Autodesk Inventor part; units mm, degrees
ref_plane "YZ Plane" through (0, 0, 0) normal (1, 0, 0) x (0, 1, 0)
ref_plane "XZ Plane" through (0, 0, 0) normal (0, 1, 0) x (-1, 0, 0)
ref_plane "XY Plane" through (0, 0, 0) normal (0, 0, 1) x (1, 0, 0)
sketch "Эскиз1" plane through (0, 0, 0) normal (0, 0, 1) x (1, 0, 0)
  line L0 (0, 0) -> (68, 0)
  line L1 (68, 0) -> (68, 35)
  line L2 (68, 35) -> (0, 35)
  line L3 (0, 35) -> (0, 0)
  line L4 (5, 30) -> (63, 30)
  line L5 (63, 30) -> (63, 3)
  line L6 (63, 3) -> (5, 3)
  line L7 (5, 3) -> (5, 30)
  line L8 (5, 3) -> (0, 3)
  line L9 (63, 3) -> (68, 3)
  dimension "d0" = 5
  dimension "d1" = 5
  dimension "d2" = 5
  dimension "d3" = 3
  dimension "d4" = 68
  dimension "d5" = 35
extrude "Выдавливание1" add sketch "Эскиз1" along normal blind 3 contours L3 L2 L1 L9 L5 L4 L7 L8
extrude "Выдавливание2" add sketch "Эскиз1" along normal blind 25 contours L3 L8 L6 L9 L1 L0
sketch "Эскиз2" plane through (0, 0, 0) normal (0, -1, 0) x (1, 0, 0)
  circle A0 centre (34, 12.5) radius 1
  line L0 (0, 0) -> (0, 25)
  line L1 (0, 25) -> (68, 25)
  point P0 (0, 12.5)
  point P1 (34, 25)
  dimension "d10" = 2
extrude "Выдавливание3" cut sketch "Эскиз2" against normal up to next
sketch "Эскиз3" plane through (5, 3, 0) normal (0, 1, 0) x (1, 0, 0)
  line L0 (-5, -25) -> (63, -25)
  line L1 (-5, -3) -> (-5, -25)
  line L2 (-5, -25) -> (63, -25)
  line L3 (63, -25) -> (63, -3)
  line L4 (63, -3) -> (60, -3)
  line L5 (60, -3) -> (60, -22)
  line L6 (60, -22) -> (-2, -22)
  line L7 (-2, -22) -> (-2, -3)
  line L8 (-2, -3) -> (-5, -3)
  line L9 (58, -3) -> (63, -3)
  point P0 (-5, 0)
  point P1 (60.5, -3)
  dimension "d13" = 3
  dimension "d14" = 3
  dimension "d15" = 3
extrude "Выдавливание4" add sketch "Эскиз3" along normal blind 2
properties part number "креплениедлякамерыниз"
Can you work these out from the model? Positions are in its coordinate system, mm. A direction names the side the tool comes from. Give positions to 0.01 mm unless a question says otherwise; leave off trailing zeros. Loops run counter-clockwise (first coordinate to the right, second up) from the corner with the lowest first, then second, coordinate; pieces in that order, holes last. Notation, with made-up numbers: M -30.5,35.5 L 5.5,35.5 A34 ccw 5.5,72.5 Z; hole C 37.5,-38 d6. An arc over 180 degrees is marked long. Answer in a Markdown table with one row per item.
1. Suppose I cut it at A-A on y = 7. Write out the boundary of the cut face in (x, z).
Taken from the geometry:
| item | result |
|---|---|
| outline | M 0,0 L 5,0 L 5,3 L 0,3 Z; M 63,0 L 68,0 L 68,3 L 63,3 Z |
2. For pin 1 Ø2.5 at (x, z) = (34, 12.5) entering from +Y, with a flat end and sliding along its axis, tell me the tip position at first contact or that it passes through.
Taken from the geometry:
| item | result |
|---|---|
| pin 1 | stops at y = 3 |
3. Suppose I cut it at C-C on x = 11. Write out the boundary of the cut face in (y, z).
Taken from the geometry:
| item | result |
|---|---|
| outline | M 0,0 L 3,0 L 3,22 L 5,22 L 5,25 L 0,25 Z; M 30,0 L 35,0 L 35,3 L 30,3 Z |
4. Suppose I cut it at B-B on z = 12.5. Write out the boundary of the cut face in (x, y), plus the area to 3 significant figures.
Taken from the geometry:
| item | result |
|---|---|
| outline | M 0,0 L 33,0 L 33,3 L 3,3 L 3,5 L 0,5 Z; M 35,0 L 68,0 L 68,5 L 65,5 L 65,3 L 35,3 Z |
| area | 210 mm² |
5. Suppose I cut it at D-D on x = 34. Write out the boundary of the cut face in (y, z).
Taken from the geometry:
| item | result |
|---|---|
| outline | M 0,0 L 3,0 L 3,11.5 L 0,11.5 Z; M 0,13.5 L 3,13.5 L 3,22 L 5,22 L 5,25 L 0,25 Z; M 30,0 L 35,0 L 35,3 L 30,3 Z |
6. Thinking about a two-plate mould opening in Z: for faces 1 (the cylindrical face through (33.783, 1.479, 11.524)), 2 (the flat face through (34, 2, 0)), 3 (the flat face through (63, 17, 1)), 4 (the flat face through (34, 2, 25)), which applies, released by +Z, released by -Z, zero draft, split by the parting line, or undercut?
Taken from the geometry:
| item | result |
|---|---|
| face 1 | undercut |
| face 2 | released by -Z |
| face 3 | zero draft |
| face 4 | released by +Z |
7. If I drill on line 1 along X through (y, z) = (3.5, 3.5); line 2 along Z through (x, y) = (34, 1); line 3 along Y through (x, z) = (56, 6.25), over which ranges is the centre line in solid material (lowest first)?
Taken from the geometry:
| item | result |
|---|---|
| line 1 | x = 0 to 3, 65 to 68 |
| line 2 | z = 0 to 11.5, 13.5 to 25 |
| line 3 | y = 0 to 3 |
8. Which directions (+Z, -Z, +X, -X, +Y, -Y) give clear straight access to the entire face, cutting with the end or side of a thin tool? Please do faces 5 (the flat face through (34, 5, 23)), 6 (the flat face through (3, 4, 13)), 7 (the flat face through (34, 30, 1)).
Taken from the geometry:
| item | result |
|---|---|
| face 5 | +Z, +X, -X, +Y |
| face 6 | +Y |
| face 7 | +Z, -Z |
